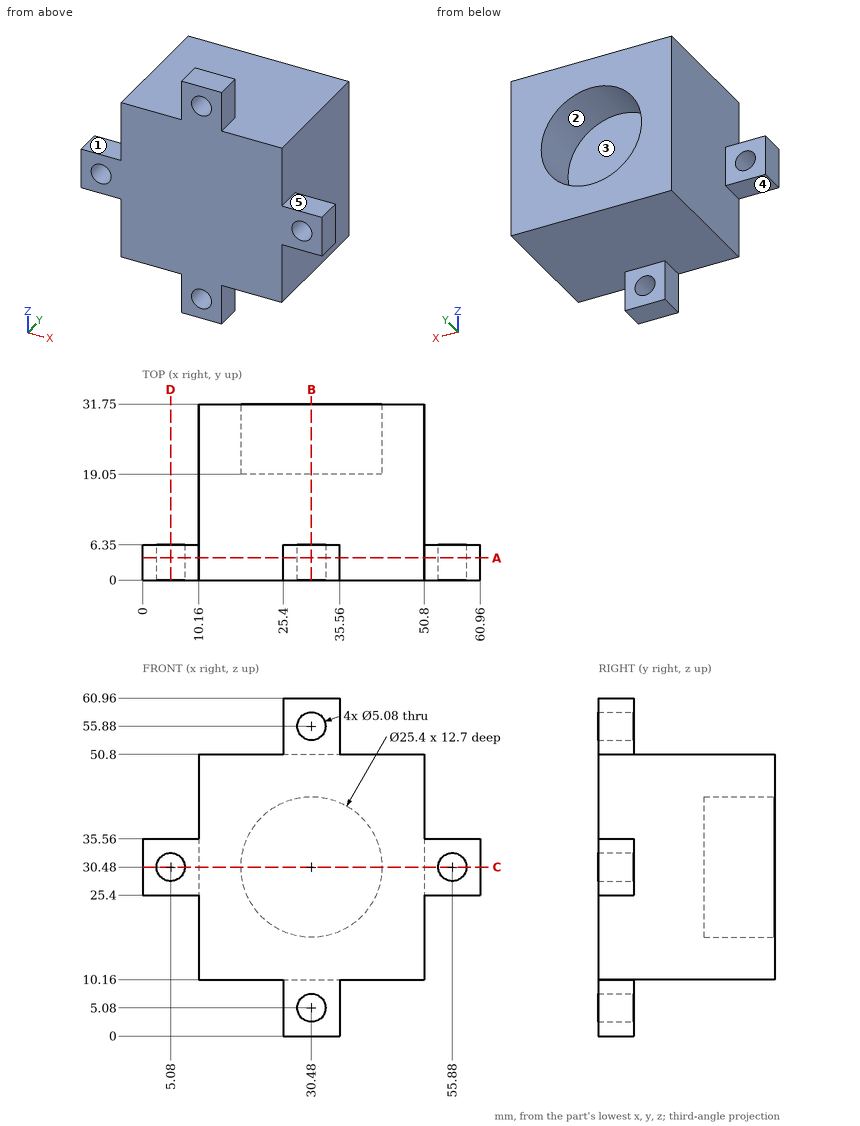
Can you work these out from the drawing? Everything is in mm from the part's minimum corner. A direction names the side the tool comes from. Coordinates: 2 decimals unless noted, no trailing zeros. Loops run counter-clockwise (first coordinate to the right, second up) from the corner with the lowest first, then second, coordinate; pieces in that order, holes last. Notation, with made-up numbers: (-23.5, 55.25) - (3.5, 55.25) arc R25 cw to (3.5, 83.25) - close; hole circle Ø11 at (86.25, -22.5). An arc over 180 degrees is marked (long way). Put each result on its own line as item: value. Start each with the question number.
Item 1: If I drill on line 1 along Z through (x, y) = (30.48, 4.25); line 2 along Z through (x, y) = (56, 3), over which ranges is the centre line in solid material (lowest first)?
Item 2: If we mould it in two halves opening along X, with no side actions, what happens to the marked faces 1 and 2? For each: +X half, -X half, draft (parallel to the pull), parting line (faces both ways), or undercut.
Item 3: Suppose I cut it at D-D (x = 5.08). Please give me the cut outline in (y, z), and give its area (3 significant figures).
Item 4: Suppose I cut it at B-B (x = 30.48). Please give me the cut outline in (y, z).
Item 5: Which directions (+Z, -Z, +X, -X, +Y, -Y) give clear straight access to the entire face, cutting with the end or side of a thin tool? Please do the marked faces 3, 4 and 5.
Item 6: Suppose I cut it at A-A (y = 4). Please give me the cut outline in (x, z), and give its area (3 significant figures).
Item 7: Suppose I cut it at C-C (z = 30.48). Please give me the cut outline in (x, y), and give its area (3 significant figures).
Item 8: For pin 1 (5 mm diameter, centred on x = 55, y = 2.5, fed in from +Z); pin 2 (8 mm diameter, centred on y = 27.5, z = 51, fed in from +X); pin 3 (9.5 mm diameter, centred on x = 37.5, y = 23.5, fed in from +Z); pin 4 (3 mm diameter, centred on x = 55.88, z = 30.48, fed in from +Y), each with a flat end and sliding along its axis, tell me the tip position at first contact or that it passes through.
Here are the results:
1. line 1: 0 to 2.54, 7.62 to 53.34, 58.42 to 60.96
1. line 2: 25.4 to 27.94, 33.02 to 35.56
2. face 1: draft
2. face 2: undercut
3. outline: (0, 25.4) - (6.35, 25.4) - (6.35, 27.94) - (0, 27.94) - close; (0, 33.02) - (6.35, 33.02) - (6.35, 35.56) - (0, 35.56) - close
3. area: 32.3 mm²
4. outline: (0, 0) - (6.35, 0) - (6.35, 2.54) - (0, 2.54) - close; (0, 7.62) - (6.35, 7.62) - (6.35, 10.16) - (31.75, 10.16) - (31.75, 17.78) - (19.05, 17.78) - (19.05, 43.18) - (31.75, 43.18) - (31.75, 50.8) - (6.35, 50.8) - (6.35, 53.34) - (0, 53.34) - close; (0, 58.42) - (6.35, 58.42) - (6.35, 60.96) - (0, 60.96) - close
5. face 3: +Y
5. face 4: -Z, -X, +Y, -Y
5. face 5: +Z, +X, +Y, -Y
6. outline: (0, 25.4) - (10.16, 25.4) - (10.16, 10.16) - (25.4, 10.16) - (25.4, 0) - (35.56, 0) - (35.56, 10.16) - (50.8, 10.16) - (50.8, 25.4) - (60.96, 25.4) - (60.96, 35.56) - (50.8, 35.56) - (50.8, 50.8) - (35.56, 50.8) - (35.56, 60.96) - (25.4, 60.96) - (25.4, 50.8) - (10.16, 50.8) - (10.16, 35.56) - (0, 35.56) - close; hole circle Ø5.08 at (5.08, 30.48); hole circle Ø5.08 at (30.48, 5.08); hole circle Ø5.08 at (30.48, 55.88); hole circle Ø5.08 at (55.88, 30.48)
6. area: 1,980 mm²
7. outline: (0, 0) - (2.54, 0) - (2.54, 6.35) - (0, 6.35) - close; (7.62, 0) - (53.34, 0) - (53.34, 6.35) - (50.8, 6.35) - (50.8, 31.75) - (43.18, 31.75) - (43.18, 19.05) - (17.78, 19.05) - (17.78, 31.75) - (10.16, 31.75) - (10.16, 6.35) - (7.62, 6.35) - close; (58.42, 0) - (60.96, 0) - (60.96, 6.35) - (58.42, 6.35) - close
7. area: 1,030 mm²
8. pin 1: z = 35.56
8. pin 2: x = 50.8
8. pin 3: z = 50.8
8. pin 4: through
